Can you work these out from the model? Positions are in its coordinate system, mm. Give positions to 0.01 mm unless a question says otherwise; leave off trailing zeros. Order: outer loops, then holes, each group sorted by start corner. A loop starts at its lowest first (then second) coordinate and runs counter-clockwise, first axis right, second up. Notation, with made-up numbers: (-5, 43.5) - (53, 43.5) arc R16 ccw to (53, 52.5) - close; hole circle Ø3 at (60, -28). An arc over 180 degrees is marked (long way). Write each question's results on one line, items separated by ' | '. Start each with the question number.
Autodesk Inventor part; units mm, degrees
ref_plane "YZ Plane" through (0, 0, 0) normal (1, 0, 0) x (0, 1, 0)
ref_plane "XZ Plane" through (0, 0, 0) normal (0, 1, 0) x (-1, 0, 0)
ref_plane "XY Plane" through (0, 0, 0) normal (0, 0, 1) x (1, 0, 0)
sketch "Sketch1" plane through (0, 0, 0) normal (0, 0, 1) x (1, 0, 0)
  line L0 (0, 0) -> (50.8, 19.05)
  line L1 (50.8, 19.05) -> (76.2, 19.05)
  line L2 (76.2, 19.05) -> (76.2, -76.2)
  line L3 (76.2, -76.2) -> (50.8, -76.2)
  line L4 (50.8, -76.2) -> (0, -25.4)
  line L5 (0, -25.4) -> (0, 0)
  line L6 (76.2, -6.35) -> (26.8732, -6.35) construction
  line L7 (26.8732, -6.35) -> (26.8732, -41.7576) construction
  line L8 (26.8732, -41.7576) -> (76.2, -41.7576) construction
  line L9 (76.2, -41.7576) -> (76.2, -6.35) construction
  circle A0 centre (33.8732, -13.65) radius 2.3813
  circle A1 centre (66.0064, -13.65) radius 2.3813
  circle A2 centre (33.8732, -34.4576) radius 2.3813
  circle A3 centre (66.0064, -34.4576) radius 2.3813
  line L10 (0, 0) -> (76.2, 0) construction
  circle A4 centre (12.7, -12.7) radius 3.175
  circle A5 centre (63.5, -63.5) radius 3.175
  circle A6 centre (63.5, 6.35) radius 3.175
  dimension "d0" = 25.4
  dimension "d1" = 95.25
  dimension "d2" = 19.05
  dimension "d3" = 76.2
  dimension "d4" = 25.4
  dimension "d5" = 25.4
  dimension "d6" = 49.3268
  dimension "d7" = 35.4076
  dimension "d8" = 25.4
  dimension "d9" = 4.7625
  dimension "d10" = 7.3
  dimension "d11" = 7.3
  dimension "d12" = 7.3
  dimension "d13" = 7.3
  dimension "d14" = 10.1936
  dimension "d15" = 10.1936
  dimension "d16" = 7
  dimension "d17" = 7
  dimension "d18" = 6.35
  dimension "d19" = 12.7
  dimension "d20" = 12.7
  dimension "d21" = 6.35
  dimension "d22" = 6.35
  dimension "d23" = 12.7
  dimension "d24" = 12.7
  dimension "d25" = 12.7
  dimension "d26" = 12.7
extrude "Extrusion1" add sketch "Sketch1" along normal blind 3.175
properties part number "15102898-16-P-0309" material "Aluminum 6061"
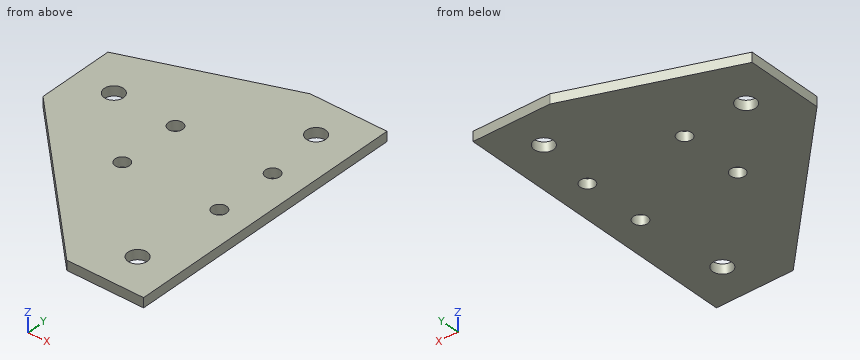
Q1. Will these pins go through, and if not, where does the flat tip stop? P1, Ø5.5, axis at x = 63.5, y = 6.35, coming from the +Z side; P2, Ø1, axis at x = 21.5, z = 1, coming from the +Y side.
Q2. If we section it at B-B (x = 12.7): Please give me the cut outline in (y, z) (1 decimal).
Q3. If I drill on probe 1 along Y at (x, z) = (33, 0.75) (3 decimals); probe 2 along Y at (x, z) = (36, 2.7); probe 3 along Y at (x, z) = (12, 1.8), over which ranges is the centre line in solid material (lowest first)? Write a range as from..to.
Q4. If we section it at A-A (y = -63.5): Please give me the cut outline in (x, z) (3 decimals), plus the area to 3 significant figures.
Q5. If we section it at D-D (y = -49.5): Please give me the cut outline in (x, z) (3 decimals), plus the area to 3 significant figures.
Q6. If we section it at C-C (z = 1.5): State how many separate pieces and enclosed holes the cut face has, plus the area to 3 significant figures.
Findings below:
1) P1: passes through | P2: stops at y = 8.25
2) outline: (-38.1, 0) - (-15.9, 0) - (-15.9, 3.2) - (-38.1, 3.2) - close; (-9.5, 0) - (4.8, 0) - (4.8, 3.2) - (-9.5, 3.2) - close
3) probe 1: y = -58.4..-36.673, -32.242..-15.865, -11.435..12.375 | probe 2: y = -61.4..-35.53, -33.39..-14.72, -12.58..13.5 | probe 3: y = -37.4..-15.8, -9.6..4.5
4) outline: (38.1, 0) - (60.325, 0) - (60.325, 3.175) - (38.1, 3.175) - close; (66.675, 0) - (76.2, 0) - (76.2, 3.175) - (66.675, 3.175) - close | area: 101 mm2
5) outline: (24.1, 0) - (76.2, 0) - (76.2, 3.175) - (24.1, 3.175) - close | area: 165 mm2
6) separate pieces: 1 | enclosed holes: 7 | area: 5,320 mm2
